from build123d import *

# Parameters (mm, degrees)
F0_W      = 70
F0_H      = 130
F0_R      = 2.25
F1_DEPTH  = 8
F3_W      = 13
F3_H      = 24
F4_DEPTH  = 30
F5_R      = 1.8965654334
F5_R_2    = 5.25
F6_DEPTH  = 41.501
F7_R      = 2.75
F8_DEPTH  = 8.001
F9_R      = 5
F9_R_2    = 2.75
F10_DEPTH = 5
F11_W     = 13
F11_H     = 30
F12_DEPTH = 4
F13_W     = 13
F13_H     = 30
F14_DEPTH = 4
F15_R     = 3.75
F15_R_2   = 2.25
F16_DEPTH = 5
F17_DEPTH = 4
F18_DEPTH = 4


# Not quite as in the source:
# - a feature names something its author has since deleted; it is built from what else it names


with BuildPart() as f1:
    # F0 (on Front) → F1 (new body)
    with BuildSketch(Plane.XZ):
        with Locations((35, 65)):
            Rectangle(F0_W, F0_H)
        with Locations((6, 4.8520950079)):
            Circle(F0_R, mode=Mode.SUBTRACT)
        with Locations((6, 28.8520950079)):
            Circle(F0_R, mode=Mode.SUBTRACT)
        with Locations((24, 4.8520950079)):
            Circle(F0_R, mode=Mode.SUBTRACT)
        with Locations((24, 28.8520950079)):
            Circle(F0_R, mode=Mode.SUBTRACT)
        with Locations((46, 4.8520950079)):
            Circle(F0_R, mode=Mode.SUBTRACT)
        with Locations((46, 28.8520950079)):
            Circle(F0_R, mode=Mode.SUBTRACT)
        with Locations((64, 4.8520950079)):
            Circle(F0_R, mode=Mode.SUBTRACT)
        with Locations((64, 28.8520950079)):
            Circle(F0_R, mode=Mode.SUBTRACT)
        with Locations((6, 101.1479049921)):
            Circle(F0_R, mode=Mode.SUBTRACT)
        with Locations((6, 125.1479049921)):
            Circle(F0_R, mode=Mode.SUBTRACT)
        with Locations((24, 101.1479049921)):
            Circle(F0_R, mode=Mode.SUBTRACT)
        with Locations((24, 125.1479049921)):
            Circle(F0_R, mode=Mode.SUBTRACT)
        with Locations((46, 101.1479049921)):
            Circle(F0_R, mode=Mode.SUBTRACT)
        with Locations((46, 125.1479049921)):
            Circle(F0_R, mode=Mode.SUBTRACT)
        with Locations((64, 101.1479049921)):
            Circle(F0_R, mode=Mode.SUBTRACT)
        with Locations((64, 125.1479049921)):
            Circle(F0_R, mode=Mode.SUBTRACT)
    extrude(amount=-F1_DEPTH)

    # F3 (on face) → F4 (join)
    with BuildSketch(Plane(origin=(0, 8, 0), x_dir=(-1, 0, 0), z_dir=(0, 1, 0))):
        with Locations((-35, 65)):
            Rectangle(F3_W, F3_H)
    extrude(amount=F4_DEPTH)

    # F5 (on face) → F6 (cut, through all)
    with BuildSketch(Plane(origin=(28.5, 0, 0), x_dir=(0, -1, 0), z_dir=(-1, 0, 0))):
        with Locations((-32, 65)):
            Circle(F5_R)
        with Locations((-24, 73)):
            Circle(F5_R)
        with Locations((-16, 65)):
            Circle(F5_R)
        with Locations((-24, 57)):
            Circle(F5_R)
        with Locations((-24, 65)):
            Circle(F5_R_2)
    extrude(amount=-F6_DEPTH, mode=Mode.SUBTRACT)

    # F7 (on face) → F8 (cut, through all)
    with BuildSketch(Plane(origin=(0, 8, 0), x_dir=(-1, 0, 0), z_dir=(0, 1, 0))):
        with Locations((-60, 90)):
            Circle(F7_R)
        with Locations((-10, 90)):
            Circle(F7_R)
        with Locations((-60, 40)):
            Circle(F7_R)
        with Locations((-10, 40)):
            Circle(F7_R)
    extrude(amount=-F8_DEPTH, mode=Mode.SUBTRACT)

    # F9 (on face) → F10 (cut)
    with BuildSketch(Plane(origin=(0, 8, 0), x_dir=(-1, 0, 0), z_dir=(0, 1, 0))):
        with Locations((-60, 90)):
            Circle(F9_R)
        with Locations((-60, 90)):
            Circle(F9_R_2, mode=Mode.SUBTRACT)
        with Locations((-10, 90)):
            Circle(F9_R)
        with Locations((-10, 90)):
            Circle(F9_R_2, mode=Mode.SUBTRACT)
        with Locations((-10, 40)):
            Circle(F9_R)
        with Locations((-10, 40)):
            Circle(F9_R_2, mode=Mode.SUBTRACT)
        with Locations((-60, 40)):
            Circle(F9_R)
        with Locations((-60, 40)):
            Circle(F9_R_2, mode=Mode.SUBTRACT)
    extrude(amount=-F10_DEPTH, mode=Mode.SUBTRACT)

    # F11 (on face) → F12 (join)
    with BuildSketch(Plane.XY.offset(77)):
        with Locations((35, 23)):
            Rectangle(F11_W, F11_H)
    extrude(amount=F12_DEPTH)

    # F13 (on face) → F14 (join)
    with BuildSketch(Plane(origin=(0, 0, 53), x_dir=(1, 0, 0), z_dir=(0, 0, -1))):
        with Locations((35, -23)):
            Rectangle(F13_W, F13_H)
    extrude(amount=F14_DEPTH)

    # F15 (on face) → F16 (cut)
    with BuildSketch(Plane.XZ):
        with Locations((6, 125.1479049921)):
            Circle(F15_R)
        with Locations((6, 125.1479049921)):
            Circle(F15_R_2, mode=Mode.SUBTRACT)
        with Locations((24, 101.1479049921)):
            Circle(F15_R)
        with Locations((24, 101.1479049921)):
            Circle(F15_R_2, mode=Mode.SUBTRACT)
        with Locations((24, 125.1479049921)):
            Circle(F15_R)
        with Locations((24, 125.1479049921)):
            Circle(F15_R_2, mode=Mode.SUBTRACT)
        with Locations((6, 101.1479049921)):
            Circle(F15_R)
        with Locations((6, 101.1479049921)):
            Circle(F15_R_2, mode=Mode.SUBTRACT)
        with Locations((46, 125.1479049921)):
            Circle(F15_R)
        with Locations((46, 125.1479049921)):
            Circle(F15_R_2, mode=Mode.SUBTRACT)
        with Locations((64, 125.1479049921)):
            Circle(F15_R)
        with Locations((64, 125.1479049921)):
            Circle(F15_R_2, mode=Mode.SUBTRACT)
        with Locations((46, 101.1479049921)):
            Circle(F15_R)
        with Locations((46, 101.1479049921)):
            Circle(F15_R_2, mode=Mode.SUBTRACT)
        with Locations((64, 101.1479049921)):
            Circle(F15_R)
        with Locations((64, 101.1479049921)):
            Circle(F15_R_2, mode=Mode.SUBTRACT)
        with Locations((6, 28.8520950079)):
            Circle(F15_R)
        with Locations((6, 28.8520950079)):
            Circle(F15_R_2, mode=Mode.SUBTRACT)
        with Locations((24, 28.8520950079)):
            Circle(F15_R)
        with Locations((24, 28.8520950079)):
            Circle(F15_R_2, mode=Mode.SUBTRACT)
        with Locations((46, 28.8520950079)):
            Circle(F15_R)
        with Locations((46, 28.8520950079)):
            Circle(F15_R_2, mode=Mode.SUBTRACT)
        with Locations((6, 4.8520950079)):
            Circle(F15_R)
        with Locations((6, 4.8520950079)):
            Circle(F15_R_2, mode=Mode.SUBTRACT)
        with Locations((64, 28.8520950079)):
            Circle(F15_R)
        with Locations((64, 28.8520950079)):
            Circle(F15_R_2, mode=Mode.SUBTRACT)
        with Locations((24, 4.8520950079)):
            Circle(F15_R)
        with Locations((24, 4.8520950079)):
            Circle(F15_R_2, mode=Mode.SUBTRACT)
        with Locations((46, 4.8520950079)):
            Circle(F15_R)
        with Locations((46, 4.8520950079)):
            Circle(F15_R_2, mode=Mode.SUBTRACT)
        with Locations((64, 4.8520950079)):
            Circle(F15_R)
        with Locations((64, 4.8520950079)):
            Circle(F15_R_2, mode=Mode.SUBTRACT)
    extrude(amount=-F16_DEPTH, mode=Mode.SUBTRACT)

    # F13 (on face) → F17 (join)
    with BuildSketch(Plane(origin=(0, 0, 53), x_dir=(1, 0, 0), z_dir=(0, 0, -1))):
        with BuildLine():
            Line((52.5, -8), (52.4993246093, -8))
            Line((52.4993246093, -8), (41.5, -8))
            Line((41.5, -8), (41.5, -38))
            Line((41.5, -38), (47.5, -38))
            ThreePointArc((47.5, -38), (51.0355339059, -36.5355339059), (52.5, -33))
            Line((52.5, -33), (52.5, -8))
        make_face()
        with BuildLine():
            Line((28.5, -38), (28.5, -8))
            Line((28.5, -8), (17.5, -8))
            Line((17.5, -8), (17.5, -33))
            ThreePointArc((17.5, -33), (18.9644660941, -36.5355339059), (22.5, -38))
            Line((22.5, -38), (28.5, -38))
        make_face()
    extrude(amount=F17_DEPTH)

    # F11 (on face) → F18 (join)
    with BuildSketch(Plane.XY.offset(77)):
        with BuildLine():
            Line((28.5, 8), (28.5, 38))
            Line((28.5, 38), (22.5, 38))
            ThreePointArc((22.5, 38), (18.9644660941, 36.5355339059), (17.5, 33))
            Line((17.5, 33), (17.5, 8))
            Line((17.5, 8), (28.5, 8))
        make_face()
        with BuildLine():
            Line((47.5, 38), (41.5, 38))
            Line((41.5, 38), (41.5, 8))
            Line((41.5, 8), (52.5, 8))
            Line((52.5, 8), (52.5, 33))
            ThreePointArc((52.5, 33), (51.0355339059, 36.5355339059), (47.5, 38))
        make_face()
        with Locations((35, 23)):
            Rectangle(F11_W, F11_H)
    extrude(amount=F18_DEPTH)


solid = f1.part
Verification items for the finished model (mm, model axes). A direction names the side the tool comes from. Round coordinates to 2 decimals unless told otherwise and drop trailing zeros. Write each loop counter-clockwise with the first axis right and the second up, starting at its lowest first coordinate (ties: lowest second). Pieces come first, ordered by that corner, then holes.
(1) Section check C-C (x = 24). Give the number of separate pieces and of enclosed holes in the cut face, plus the area to 3 significant figures.
Returned:
separate pieces: 5
enclosed holes: 0
area: 1,080 mm2
(2) Section check D-D (z = 118.5). Enter the section's corners in (x, y), plus the area to 3 significant figures.
Returned:
outline: (0, 0) - (70, 0) - (70, 8) - (0, 8) - close
area: 560 mm2
(3) Access from +Z, -Z, +X, -X, +Y, -Y to the whole of each face (thin tool, end or side, straight path). Record for faces 1 (the cylindrical face through (43.752, 6.479, 4.951)), 2 (the flat face through (8.4, 5, 101.2)), 3 (the flat face through (7.8, 3, 37.8)), 4 (the flat face through (28.5, 23, 71)).
Returned:
face 1: +Y, -Y
face 2: -Y
face 3: +Y
face 4: -X, +Y
(4) Section check B-B (z = 65). Enter the section's corners in (x, y).
Returned:
outline: (0, 0) - (70, 0) - (70, 8) - (41.5, 8) - (41.5, 14.1) - (28.5, 14.1) - (28.5, 8) - (0, 8) - close; (28.5, 17.9) - (41.5, 17.9) - (41.5, 18.75) - (28.5, 18.75) - close; (28.5, 29.25) - (41.5, 29.25) - (41.5, 30.1) - (28.5, 30.1) - close; (28.5, 33.9) - (41.5, 33.9) - (41.5, 38) - (28.5, 38) - close
(5) Mould release check, pull along Z, two halves, no side actions. Record for faces 5 (the flat face through (0, 4, 64)), 6 (the cylindrical face through (25.21, 6.48, 30.75)): pulls with the +Z half, pulls with the -Z half, needs draft (parallel to the pull), parting line crosses it, or undercut.
Returned:
face 5: needs draft
face 6: undercut
(6) Section check A-A (y = 24). Enter the section's corners in (x, z), plus the area to 3 significant figures.
Returned:
outline: (17.5, 49) - (52.5, 49) - (52.5, 53) - (41.5, 53) - (41.5, 55.1) - (28.5, 55.1) - (28.5, 53) - (17.5, 53) - close; (17.5, 77) - (28.5, 77) - (28.5, 74.9) - (41.5, 74.9) - (41.5, 77) - (52.5, 77) - (52.5, 81) - (17.5, 81) - close; (28.5, 58.9) - (41.5, 58.9) - (41.5, 59.75) - (28.5, 59.75) - close; (28.5, 70.25) - (41.5, 70.25) - (41.5, 71.1) - (28.5, 71.1) - close
area: 357 mm2
(7) Depth check by flat-ended pin: pin 1 Ø12 at (x, z) = (46, 28.85) entering from +Y; pin 2 Ø5 at (x, z) = (64, 28.85) entering from -Y; pin 3 Ø5 at (x, z) = (61.5, 41) entering from +Y. Enter the tip coordinate at first touch or a pass-through.
Returned:
pin 1: stops at y = 8
pin 2: stops at y = 5
pin 3: stops at y = 3
(8) Material ranges on line 1 (Z direction, x = 10, y = 5); line 2 (Z direction, x = 60, y = 2); line 3 (Z direction, x = 34, y = 24), recorded low to high.
Returned:
line 1: z = 0 to 35, 45 to 85, 95 to 130
line 2: z = 0 to 37.25, 42.75 to 87.25, 92.75 to 130
line 3: z = 49 to 55.1, 58.9 to 59.75, 70.25 to 71.1, 74.9 to 81
